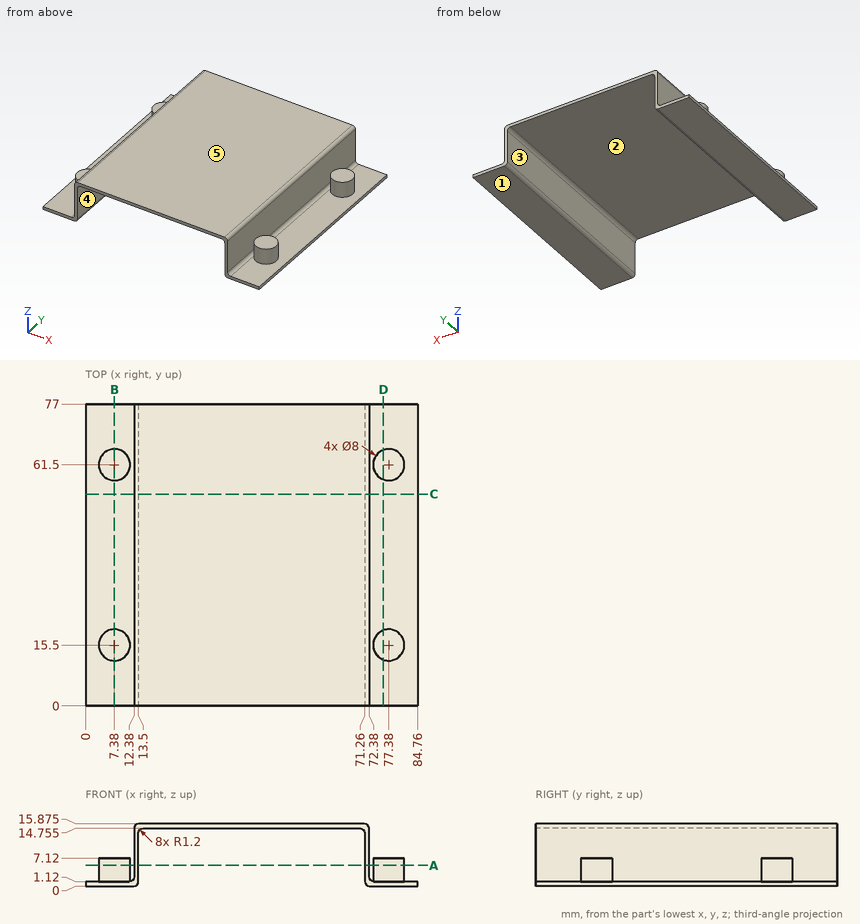
Design review of the part shown in the three views and the two pictorial views. Dimensions are in mm from the part's minimum x, y and z. A direction names the side the tool comes from. Round coordinates to 2 decimals unless told otherwise and drop trailing zeros. Order: outer loops, then holes, each group sorted by start corner. A loop starts at its lowest first (then second) coordinate and runs counter-clockwise, first axis right, second up. Notation, with made-up numbers: (52.25, -11.75) - (79.25, -11.75) arc R21 cw to (79.25, 8.25) - close; hole circle Ø7 at (-18.75, 45.25). An arc over 180 degrees is marked (long way). Answer in a Markdown table with one row per item.
(1) Take a section at D-D on x = 76. Write out the cut boundary in (y, z).
Result set:
| item | result |
|---|---|
| outline | (0, 0) - (77, 0) - (77, 1.12) - (65.25, 1.12) - (65.25, 7.12) - (57.75, 7.12) - (57.75, 1.12) - (19.25, 1.12) - (19.25, 7.12) - (11.75, 7.12) - (11.75, 1.12) - (0, 1.12) - close |
(2) Take a section at A-A on z = 5.25. Write out the cut boundary in (x, y), plus the area to 3 significant figures.
Result set:
| item | result |
|---|---|
| outline | circle Ø8 at (7.38, 15.5); circle Ø8 at (7.38, 61.5); (12.38, 0) - (13.5, 0) - (13.5, 77) - (12.38, 77) - close; (71.26, 0) - (72.38, 0) - (72.38, 77) - (71.26, 77) - close; circle Ø8 at (77.38, 15.5); circle Ø8 at (77.38, 61.5) |
| area | 374 mm2 |
(3) Clearance check with flat-ended pins moving along their axes: P1, Ø6, axis at y = 35.5, z = 11, coming from the +X side; P2, Ø8, axis at y = 51, z = 5.5, coming from the +X side; P3, Ø9, axis at x = 5, y = 40, coming from the +Z side. State where each tip first meets the part, or that it passes through.
Result set:
| item | result |
|---|---|
| P1 | stops at x = 72.38 |
| P2 | stops at x = 72.7 |
| P3 | stops at z = 1.12 |
(4) Mouldability with a two-part tool opening along X and no side actions: class the marked faces 1, 2 and 3 as released by +X, released by -X, zero draft, split by the parting line, or undercut.
Result set:
| item | result |
|---|---|
| face 1 | zero draft |
| face 2 | undercut |
| face 3 | undercut |
(5) Machinability: for the marked faces 4 and 5, which of the approach directions +Z, -Z, +X, -X, +Y, -Y give a long, thin tool a straight path to every point of the face, cutting with its end or side? Answer none if there is none.
Result set:
| item | result |
|---|---|
| face 4 | -Z, +Y, -Y |
| face 5 | +Z, +X, -X, +Y, -Y |
(6) Take a section at B-B on x = 7.38. Write out the cut boundary in (y, z).
Result set:
| item | result |
|---|---|
| outline | (0, 0) - (77, 0) - (77, 1.12) - (65.5, 1.12) - (65.5, 7.12) - (57.5, 7.12) - (57.5, 1.12) - (19.5, 1.12) - (19.5, 7.12) - (11.5, 7.12) - (11.5, 1.12) - (0, 1.12) - close |
(7) For line 1 (X direction, y = 38.5, z = 7.25); line 2 (Z direction, x = 33, y = 69.5) (3 decimals); line 3 (X direction, y = 59.5, z = 2), list the stretches that pass through material, from the lowest coordinate up. Write a range as from..to.
Result set:
| item | result |
|---|---|
| line 1 | x = 12.38..13.5, 71.26..72.38 |
| line 2 | z = 14.755..15.875 |
| line 3 | x = 3.92..10.84, 12.34..13.5, 71.26..72.42, 73.92..80.84 |
(8) Take a section at C-C on y = 54. Write out the cut boundary in (x, z) (3 decimals).
Result set:
| item | result |
|---|---|
| outline | (0, 0) - (12.3, 0) arc R1.2 ccw to (13.5, 1.2) - (13.5, 13.555) arc R1.2 cw to (14.7, 14.755) - (70.06, 14.755) arc R1.2 cw to (71.26, 13.555) - (71.26, 1.2) arc R1.2 ccw to (72.46, 0) - (84.76, 0) - (84.76, 1.12) - (73.58, 1.12) arc R1.2 cw to (72.38, 2.32) - (72.38, 14.675) arc R1.2 ccw to (71.18, 15.875) - (13.58, 15.875) arc R1.2 ccw to (12.38, 14.675) - (12.38, 2.32) arc R1.2 cw to (11.18, 1.12) - (0, 1.12) - close |
